The figure shows three views and two pictorial views of one solid part (mm, origin at its lowest corner). Answer the questions. Give positions to 0.01 mm unless a question says otherwise; leave off trailing zeros. Order: outer loops, then holes, each group sorted by start corner. A loop starts at its lowest first (then second) coordinate and runs counter-clockwise, first axis right, second up. Notation, with made-up numbers: M 14.25,-36 L 42.25,-36 A19 ccw 42.25,-20 Z; hole C 6,42.25 d2. An arc over 180 degrees is marked long. Write item = value, one per line. Start each with the question number.
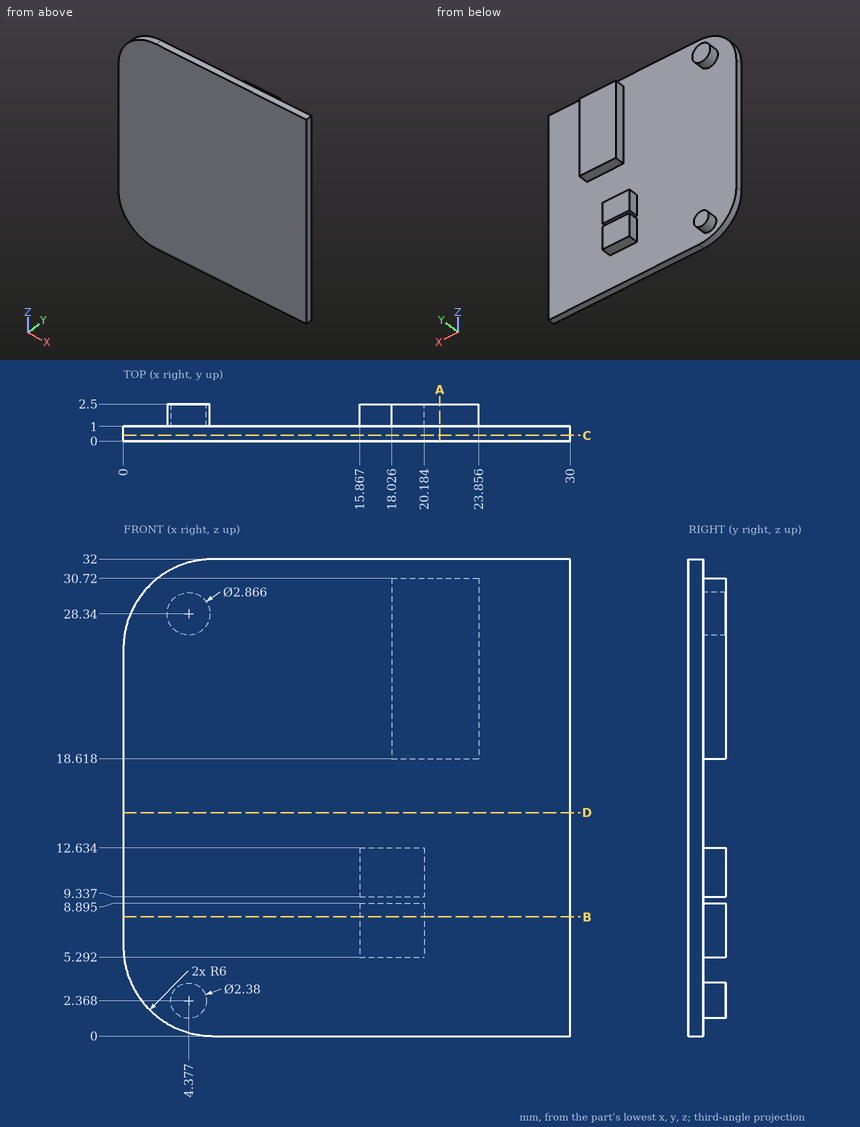
1) Each of these flat-tipped pins is pushed along its axis until it touches: P1, Ø1.2, axis at y = 2, z = 10.5, coming from the +X side; P2, Ø1.2, axis at y = 2, z = 24.5, coming from the +X side; P3, Ø0.8, axis at y = 2, z = 23.5, coming from the -X side. Where does it stop, or does it pass through?
2) Find section B-B on z = 8. Determine the outline of the cut face in (x, y) (1 decimal).
3) Find the intervals of material crossed by probe 1 along Z at (x, y) = (19.5, 1.45) (1 decimal); probe 2 along Z at (x, y) = (17, 2) (1 decimal); probe 3 along Z at (x, y) = (21.5, 2.3), in increasing order. Write a range as [from, to].
4) Find section A-A on x = 21.25. Determine the outline of the cut face in (y, z).
5) Find section D-D on z = 15. Determine the outline of the cut face in (x, y).
6) Find section C-C on y = 0.4. Determine the outline of the cut face in (x, z).
Numbers:
q1.P1 = 20.18
q1.P2 = 23.86
q1.P3 = 18.03
q2.outline = M 0,0 L 30,0 L 30,1 L 20.2,1 L 20.2,2.5 L 15.9,2.5 L 15.9,1 L 0,1 Z
q3.probe_1 = [5.3, 8.9], [9.3, 12.6], [18.6, 30.7]
q3.probe_2 = [5.3, 8.9], [9.3, 12.6]
q3.probe_3 = [18.62, 30.72]
q4.outline = M 0,0 L 1,0 L 1,18.62 L 2.5,18.62 L 2.5,30.72 L 1,30.72 L 1,32 L 0,32 Z
q5.outline = M 0,0 L 30,0 L 30,1 L 0,1 Z
q6.outline = M 0,6 A6 ccw 6,0 L 30,0 L 30,32 L 6,32 A6 ccw 0,26 Z
